Study the drawing (mm; zero at the part's minimum x, y, z) and answer. A direction names the side the tool comes from. Coordinates: 2 decimals unless noted, no trailing zeros. Write each loop counter-clockwise with the first axis right and the second up, starting at its lowest first coordinate (ties: lowest second). Pieces come first, ordered by that corner, then holes. Notation, with made-up numbers: M -2,0 L 56,0 A32 cw 56,30 Z; hole C -32,-3.5 d1. An arc over 180 degrees is marked long. Answer as CSV lines item,"result". Start each with the question number.
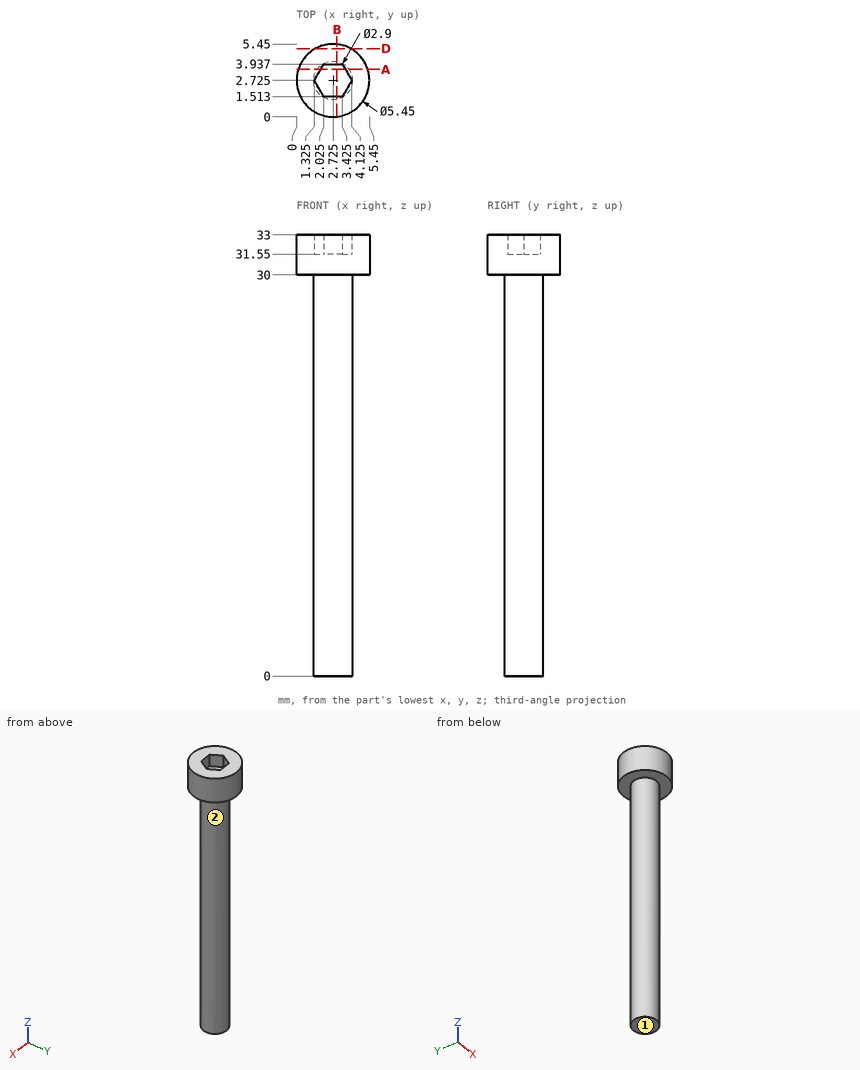
1) The part is cut by section A-A (y = 3.55). Determine the outline of the cut face in (x, z).
2) Find the intervals of material crossed by line 1 (Z direction, x = 3.6, y = 3.3); line 2 (Z direction, x = 2.15, y = 0.5); line 3 (X direction, y = 2.6, z = 24), in increasing order. Write a range as from..to.
3) The part is cut by section D-D (y = 5.1). Determine the outline of the cut face in (x, z).
4) The part is cut by section B-B (x = 3). Determine the outline of the cut face in (y, z).
5) Which of the six approach directions +Z, -Z, +X, -X, +Y, -Y give full straight-line access (tool end or side, diameter ignored) to the marked faces 1 and 2?
6) Each of these flat-tipped pins is pushed along its axis until it touches: P1, Ø1.5, axis at x = 2.5, z = 19, coming from the -Y side (3 decimals); P2, Ø1, axis at y = 3.5, z = 23, coming from the +X side; P3, Ø2, axis at y = 2.5, z = 13, coming from the -X side (3 decimals). Where does it stop, or does it pass through?
Completed:
1,outline,"M 0.13,30 L 1.53,30 L 1.53,0 L 3.92,0 L 3.92,30 L 5.32,30 L 5.32,33 L 3.65,33 L 3.65,31.55 L 1.8,31.55 L 1.8,33 L 0.13,33 Z"
2,line 1,"0..31.55"
2,line 2,"30..33"
2,line 3,"1.28..4.17"
3,outline,"M 1.39,30 L 4.06,30 L 4.06,33 L 1.39,33 Z"
4,outline,"M 0.01,30 L 1.3,30 L 1.3,0 L 4.15,0 L 4.15,30 L 5.44,30 L 5.44,33 L 3.94,33 L 3.94,31.55 L 1.51,31.55 L 1.51,33 L 0.01,33 Z"
5,face 1,"-Z, +X, -X, +Y, -Y"
5,face 2,"-Z"
6,P1,"y = 1.275"
6,P2,"x = 4.15"
6,P3,"x = 1.275"
